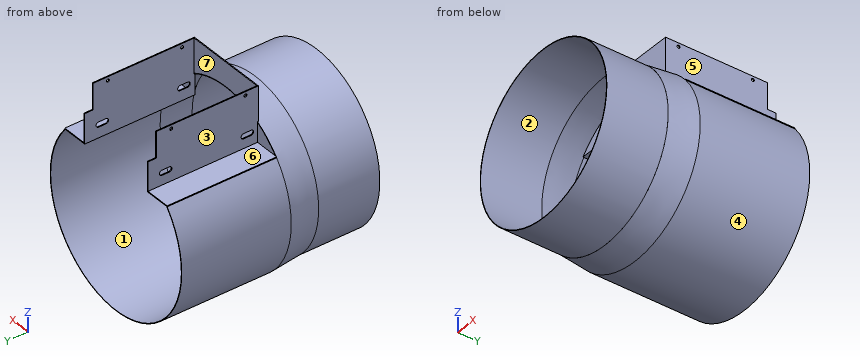
from build123d import *

# Parameters (mm, degrees)
F0_R      = 141.2875
F0_R_2    = 140.49375
F1_DEPTH  = 104.775
F6_R      = 146.558
F6_R_2    = 145.7151605206
F7_DEPTH  = 187.325
F8_W      = 355.6
F8_H      = 187.325
F9_DEPTH  = 54.484
F10_W     = 44.1738647784
F10_H     = 187.325
F11_DEPTH = 1.5875
F12_W     = 1.5875
F12_H     = 187.325
F13_DEPTH = 93.6625
F15_DEPTH = 1.5875
F17_DEPTH = 1.5875
F18_W     = 14.2875
F18_H     = 44.45
F19_DEPTH = 217.9965
F20_R     = 2.5527
F21_DEPTH = 217.9965


with BuildPart() as f1:
    # F0 (on Front) → F1 (new body)
    with BuildSketch(Plane.XZ):
        Circle(F0_R)
        Circle(F0_R_2, mode=Mode.SUBTRACT)
    extrude(amount=F1_DEPTH)

    # F3 (on Right) → F4 (revolve)
    with BuildSketch(Plane.YZ):
        Polygon((0, 141.3524150848), (0, 140.5095756054), (50.8, 145.7151605206), (50.8, 146.558), align=None)
    revolve(axis=Axis((0, 43.5656532645, 0), (0, 1, 0)))

    # F6 (on face) → F7 (join)
    with BuildSketch(Plane(origin=(0, 50.8, 0), x_dir=(-1, 0, 0), z_dir=(0, 1, 0))):
        Circle(F6_R)
        Circle(F6_R_2, mode=Mode.SUBTRACT)
    extrude(amount=F7_DEPTH)

    # F8 (on offset) → F9 (cut, through all)
    with BuildSketch(Plane.XY.offset(92.075)):
        with Locations((0, 144.4625)):
            Rectangle(F8_W, F8_H)
    extrude(amount=F9_DEPTH, mode=Mode.SUBTRACT)

    # F10 (on offset) → F11 (join)
    with BuildSketch(Plane.XY.offset(92.075)):
        with Locations((91.9369323892, 144.4625)):
            Rectangle(F10_W, F10_H)
        with Locations((-91.9369323892, 144.4625)):
            Rectangle(F10_W, F10_H)
    extrude(amount=F11_DEPTH)

    # F12 (on face) → F13 (join)
    with BuildSketch(Plane.XY.offset(93.6625)):
        with Locations((70.64375, 144.4625)):
            Rectangle(F12_W, F12_H)
        with Locations((-70.64375, 144.4625)):
            Rectangle(F12_W, F12_H)
    extrude(amount=F13_DEPTH)

    # F14 (on face) → F15 (join)
    with BuildSketch(Plane(origin=(0, 50.8, 0), x_dir=(-1, 0, 0), z_dir=(0, 1, 0))):
        with BuildLine():
            Line((69.85, 92.075), (112.5973956514, 92.075))
            ThreePointArc((112.5973956514, 92.075), (92.9351127931, 111.8885335618), (69.85, 127.5811766385))
            Line((69.85, 127.5811766385), (69.85, 92.075))
        make_face()
        with BuildLine():
            ThreePointArc((-69.85, 127.5811766385), (-92.9351127931, 111.8885335618), (-112.5973956514, 92.075))
            Line((-112.5973956514, 92.075), (-69.85, 92.075))
            Line((-69.85, 92.075), (-69.85, 127.5811766385))
        make_face()
    extrude(amount=-F15_DEPTH)

    # F16 (on face) → F17 (join)
    with BuildSketch(Plane(origin=(0, 50.8, 0), x_dir=(-1, 0, 0), z_dir=(0, 1, 0))):
        with BuildLine():
            ThreePointArc((-71.4375, 128.0071860315), (0, 146.5918008687), (71.4375, 128.0071860315))
            Line((71.4375, 128.0071860315), (71.4375, 187.325))
            Line((71.4375, 187.325), (-71.4375, 187.325))
            Line((-71.4375, 187.325), (-71.4375, 128.0071860315))
        make_face()
    extrude(amount=-F17_DEPTH)

    # F18 (on face) → F19 (cut, through all)
    with BuildSketch(Plane(origin=(-71.4375, 0, 0), x_dir=(0, -1, 0), z_dir=(-1, 0, 0))):
        with Locations((-230.98125, 165.1)):
            Rectangle(F18_W, F18_H)
    extrude(amount=-F19_DEPTH, mode=Mode.SUBTRACT)

    # F20 (on face) → F21 (cut, through all)
    with BuildSketch(Plane(origin=(-71.4375, 0, 0), x_dir=(0, -1, 0), z_dir=(-1, 0, 0))):
        with BuildLine():
            Line((-61.7855314592, 109.9362217483), (-62.0382119647, 109.936185368))
            ThreePointArc((-62.0382119647, 109.936185368), (-61.9118714487, 109.9343750452), (-61.7855314592, 109.9362217483))
        make_face()
        with BuildLine():
            Line((-74.6118714487, 109.9343750452), (-62.0382119647, 109.936185368))
            Line((-62.0382119647, 109.936185368), (-61.7855314592, 109.9362217483))
            ThreePointArc((-61.7855314592, 109.9362217483), (-57.5470865675, 114.3429791138), (-61.8714737728, 118.6654322225))
            Line((-61.8714737728, 118.6654322225), (-61.9533941249, 118.665433462))
            Line((-61.9533941249, 118.665433462), (-74.6124339459, 118.6656249995))
            ThreePointArc((-74.6124339459, 118.6656249995), (-78.9781249909, 114.2997187514), (-74.6118714487, 109.9343750452))
        make_face()
        with BuildLine():
            Line((-61.9533941249, 118.665433462), (-61.8714737728, 118.6654322225))
            ThreePointArc((-61.8714737728, 118.6654322225), (-61.9124339459, 118.6656249995), (-61.9533941249, 118.665433462))
        make_face()
        with BuildLine():
            Line((-214.0709987284, 109.9410599022), (-201.8540012716, 109.9410599022))
            ThreePointArc((-201.8540012716, 109.9410599022), (-197.2482995581, 114.188482543), (-201.6310653813, 118.665585524))
            Line((-201.6310653813, 118.665585524), (-214.3124864102, 118.665625))
            ThreePointArc((-214.3124864102, 118.665625), (-218.6764532664, 114.4208036798), (-214.5540012716, 109.9410599022))
            Line((-214.5540012716, 109.9410599022), (-214.0709987284, 109.9410599022))
        make_face()
        with BuildLine():
            ThreePointArc((-214.5540012716, 109.9410599022), (-214.3125, 109.934375), (-214.0709987284, 109.9410599022))
            Line((-214.0709987284, 109.9410599022), (-214.5540012716, 109.9410599022))
        make_face()
        with Locations((-71.4375, 180.975)):
            Circle(F20_R)
        with Locations((-198.4375, 180.975)):
            Circle(F20_R)
    extrude(amount=-F21_DEPTH, mode=Mode.SUBTRACT)


solid = f1.part
Can you work these out from the model? Positions are in its coordinate system, mm. Face numbers are marked on the shaded views. A direction names the side the tool comes from. Round coordinates to 2 decimals unless told otherwise and drop trailing zeros. Order: outer loops, then holes, each group sorted by start corner. A loop starts at its lowest first (then second) coordinate and runs counter-clockwise, first axis right, second up. Notation, with made-up numbers: (86.25, 42.5) -> (122.25, 42.5) arc R14 cw to (122.25, 68.5) -> close; hole circle Ø4 at (1, 86). An arc over 180 degrees is marked (long way). Write each question's results on one line, items separated by ' | '. Start each with the question number.
Item 1: Thinking about a two-plate mould opening in X: for the marked faces 4, 5, 6 and 7, which applies, +X half, -X half, draft (parallel to the pull), parting line (faces both ways), or undercut?
Item 2: If we section it at C-C, the plane y = -19.5: Write out the boundary of the cut face in (x, z) (1 decimal).
Item 3: If we section it at B-B, the plane x = 0: State how many separate pieces and enclosed holes the cut face has, then the cut area to 3 significant figures.
Item 4: Please list where these lines run through material, in increasing order: L1, parallel to Z at x = 0, y = -54.5; L2, parallel to X at y = 220, z = 114.5; L3, parallel to X at y = 4, z = -12.
Item 5: Will these pins go through, and if not, where does the flat tip stop? pin 1 (1 mm diameter, centred on y = -44.5, z = 66.5, fed in from +X); pin 2 (2 mm diameter, centred on y = 142.5, z = -56.5, fed in from +X); pin 3 (6 mm diameter, centred on y = 174, z = -98, fed in from -X).
Item 6: Which directions (+Z, -Z, +X, -X, +Y, -Y) give clear straight access to the entire face, cutting with the end or side of a thin tool? Please do the marked faces 1, 2 and 3.
Results:
1) face 4: parting line | face 5: +X half | face 6: draft | face 7: undercut
2) outline: circle Ø282.6 at (0, 0); hole circle Ø281 at (0, 0)
3) separate pieces: 3 | enclosed holes: 0 | area: 475 mm2
4) L1: z = -141.29 to -140.49, 140.49 to 141.29 | L2: x = -71.44 to -69.85, 69.85 to 71.44 | L3: x = -141.25 to -140.41, 140.41 to 141.25
5) pin 1: stops at x = 124.92 | pin 2: stops at x = 135.64 | pin 3: stops at x = -111.6
6) face 1: +Y | face 2: -Y | face 3: +Z, -X, +Y
